For this review, take the finished solid that the model builds, in its own axes (mm). A direction names the side the tool comes from. Give positions to 0.01 mm unless a question says otherwise; leave off trailing zeros. Write each loop counter-clockwise with the first axis right and the second up, starting at its lowest first coordinate (ties: lowest second). Pieces come first, ordered by that corner, then holes. Notation, with made-up numbers: (89, 16.25) -> (126, 16.25) arc R22 cw to (126, 31.25) -> close; hole circle Ø11 at (-30.75, 64). An arc over 180 degrees is marked (long way). Write item = value, one per line.
```python
from build123d import *

# Parameters (mm, degrees)
SKETCH1_W          = 5
SKETCH1_H          = 36
SKETCH2_R          = 3.43154
CUT_EXTRUDE1_DEPTH = 0.5
SKETCH3_R          = 3.5
CUT_EXTRUDE2_DEPTH = 31.5
CUT_EXTRUDE3_REACH = 34.284
SKETCH4_R          = 1.5
CUT_EXTRUDE4_REACH = 38.688


with BuildPart() as part:
    # Sketch1 → Revolve1 (revolve)
    with BuildSketch(Plane.XY, mode=Mode.PRIVATE) as revolve1_sk:
        with Locations((2.5, 16.5)):
            Rectangle(SKETCH1_W, SKETCH1_H)
    revolve(revolve1_sk.sketch.rotate(Axis((0, 34.5, 0), (0, -1, 0)), 270), axis=Axis((0, 34.5, 0), (0, -1, 0)))

    # Sketch2 → Cut-Extrude1 (cut)
    with BuildSketch(Plane(origin=(0, 31.6, 0), x_dir=(1, 0, 0), z_dir=(0, 1, 0))):
        with Locations(Location((0, 0, 0), (0, 0, 90))):
            Circle(SKETCH2_R)
    extrude(amount=-CUT_EXTRUDE1_DEPTH, mode=Mode.SUBTRACT)

    # Sketch3 → Cut-Extrude2 (cut)
    with BuildSketch(Plane.XZ.offset(1.5)):
        with Locations(Location((0, 0, 0), (0, 0, 90))):
            Circle(SKETCH3_R)
    extrude(amount=-CUT_EXTRUDE2_DEPTH, mode=Mode.SUBTRACT)

    # Sketch4 → Cut-Extrude3 (cut, up to next)
    with BuildSketch(Plane.XZ.offset(-30), mode=Mode.PRIVATE) as cut_extrude3_sk1:
        with Locations(Location((0, 0, 0), (0, 0, 270))):
            Circle(SKETCH4_R)
    cut_extrude3_tool1 = extrude(cut_extrude3_sk1.sketch, amount=-CUT_EXTRUDE3_REACH, mode=Mode.PRIVATE) & part.part
    add(cut_extrude3_tool1.solids().sort_by_distance((0, 30, 0))[0], mode=Mode.SUBTRACT)

    # Sketch5 → Cut-Extrude4 (cut, up to next)
    with BuildSketch(Plane(origin=(0, 34.5, 0), x_dir=(-1, 0, 0), z_dir=(0, 1, 0)), mode=Mode.PRIVATE) as cut_extrude4_sk1:
        with BuildLine():
            Line((2.430309722, 1.842849602), (1.999275165, 1.739367361))
            ThreePointArc((1.999275165, 1.739367361), (1.931766863, 1.814049831), (1.861470643, 1.886114272))
            Line((1.861470643, 1.886114272), (1.991813569, 2.309800577))
            ThreePointArc((1.991813569, 2.309800577), (1.944143169, 2.35006539), (1.895659013, 2.389346544))
            Line((1.895659013, 2.389346544), (1.503901187, 2.181921452))
            ThreePointArc((1.503901187, 2.181921452), (1.419941007, 2.237469003), (1.333931574, 2.289787448))
            Line((1.333931574, 2.289787448), (1.354813039, 2.732577836))
            ThreePointArc((1.354813039, 2.732577836), (1.298626839, 2.75972251), (1.241897077, 2.785712054))
            Line((1.241897077, 2.785712054), (0.914031566, 2.487377393))
            ThreePointArc((0.914031566, 2.487377393), (0.818895035, 2.520299768), (0.722576679, 2.549584857))
            Line((0.722576679, 2.549584857), (0.632684622, 2.98365718))
            ThreePointArc((0.632684622, 2.98365718), (0.571513009, 2.995976115), (0.51010218, 3.007041032))
            Line((0.51010218, 3.007041032), (0.26672998, 2.636542265))
            ThreePointArc((0.26672998, 2.636542265), (0.166394877, 2.64477083), (0.065819633, 2.649182473))
            Line((0.065819633, 2.649182473), (-0.129197696, 3.047262371))
            ThreePointArc((-0.129197696, 3.047262371), (-0.191511085, 3.043981522), (-0.253744312, 3.039426562))
            Line((-0.253744312, 3.039426562), (-0.397331231, 2.620043491))
            ThreePointArc((-0.397331231, 2.620043491), (-0.496560484, 2.603061214), (-0.595073102, 2.582322211))
            Line((-0.595073102, 2.582322211), (-0.882962048, 2.919396859))
            ThreePointArc((-0.882962048, 2.919396859), (-0.942501833, 2.900722375), (-1.001647117, 2.880833743))
            Line((-1.001647117, 2.880833743), (-1.03642666, 2.438917747))
            ThreePointArc((-1.03642666, 2.438917747), (-1.128315123, 2.397791689), (-1.218575206, 2.353205148))
            Line((-1.218575206, 2.353205148), (-1.581246647, 2.608094906))
            ThreePointArc((-1.581246647, 2.608094906), (-1.634271725, 2.575200173), (-1.686612749, 2.541227545))
            Line((-1.686612749, 2.541227545), (-1.61039959, 2.104545832))
            ThreePointArc((-1.61039959, 2.104545832), (-1.689173573, 2.041860093), (-1.765509747, 1.976227551))
            Line((-1.765509747, 1.976227551), (-2.180175704, 2.132916759))
            ThreePointArc((-2.180175704, 2.132916759), (-2.223354314, 2.087868673), (-2.2656023, 2.041946674))
            Line((-2.2656023, 2.041946674), (-2.083185191, 1.637937563))
            ThreePointArc((-2.083185191, 1.637937563), (-2.143895035, 1.557630919), (-2.201510819, 1.475076308))
            Line((-2.201510819, 1.475076308), (-2.642116303, 1.523719607))
            ThreePointArc((-2.642116303, 1.523719607), (-2.672735374, 1.469348706), (-2.702235725, 1.414362784))
            Line((-2.702235725, 1.414362784), (-2.425076605, 1.068411652))
            ThreePointArc((-2.425076605, 1.068411652), (-2.463907688, 0.975530065), (-2.499182869, 0.881240596))
            Line((-2.499182869, 0.881240596), (-2.938043018, 0.818781548))
            ThreePointArc((-2.938043018, 0.818781548), (-2.954178641, 0.758504156), (-2.969077742, 0.697909279))
            Line((-2.969077742, 0.697909279), (-2.614591538, 0.431753508))
            ThreePointArc((-2.614591538, 0.431753508), (-2.629103958, 0.332133069), (-2.639822068, 0.232033297))
            Line((-2.639822068, 0.232033297), (-3.049361685, 0.062396433))
            ThreePointArc((-3.049361685, 0.062396433), (-3.05, 0), (-3.049361685, -0.062396433))
            Line((-3.049361685, -0.062396433), (-2.639822068, -0.232033297))
            ThreePointArc((-2.639822068, -0.232033297), (-2.629103958, -0.332133069), (-2.614591538, -0.431753508))
            Line((-2.614591538, -0.431753508), (-2.969077742, -0.697909279))
            ThreePointArc((-2.969077742, -0.697909279), (-2.954178641, -0.758504156), (-2.938043018, -0.818781548))
            Line((-2.938043018, -0.818781548), (-2.499182869, -0.881240596))
            ThreePointArc((-2.499182869, -0.881240596), (-2.463907688, -0.975530065), (-2.425076605, -1.068411652))
            Line((-2.425076605, -1.068411652), (-2.702235725, -1.414362784))
            ThreePointArc((-2.702235725, -1.414362784), (-2.672735374, -1.469348706), (-2.642116303, -1.523719607))
            Line((-2.642116303, -1.523719607), (-2.201510819, -1.475076308))
            ThreePointArc((-2.201510819, -1.475076308), (-2.143895035, -1.557630919), (-2.083185191, -1.637937563))
            Line((-2.083185191, -1.637937563), (-2.2656023, -2.041946674))
            ThreePointArc((-2.2656023, -2.041946674), (-2.223354314, -2.087868673), (-2.180175704, -2.132916759))
            Line((-2.180175704, -2.132916759), (-1.765509747, -1.976227551))
            ThreePointArc((-1.765509747, -1.976227551), (-1.689173573, -2.041860093), (-1.61039959, -2.104545832))
            Line((-1.61039959, -2.104545832), (-1.686612749, -2.541227545))
            ThreePointArc((-1.686612749, -2.541227545), (-1.634271725, -2.575200173), (-1.581246647, -2.608094906))
            Line((-1.581246647, -2.608094906), (-1.218575206, -2.353205148))
            ThreePointArc((-1.218575206, -2.353205148), (-1.128315123, -2.397791689), (-1.03642666, -2.438917747))
            Line((-1.03642666, -2.438917747), (-1.001647117, -2.880833743))
            ThreePointArc((-1.001647117, -2.880833743), (-0.942501833, -2.900722375), (-0.882962048, -2.919396859))
            Line((-0.882962048, -2.919396859), (-0.595073102, -2.582322211))
            ThreePointArc((-0.595073102, -2.582322211), (-0.496560484, -2.603061214), (-0.397331231, -2.620043491))
            Line((-0.397331231, -2.620043491), (-0.253744312, -3.039426562))
            ThreePointArc((-0.253744312, -3.039426562), (-0.191511085, -3.043981522), (-0.129197696, -3.047262371))
            Line((-0.129197696, -3.047262371), (0.065819633, -2.649182473))
            ThreePointArc((0.065819633, -2.649182473), (0.166394877, -2.64477083), (0.26672998, -2.636542265))
            Line((0.26672998, -2.636542265), (0.51010218, -3.007041032))
            ThreePointArc((0.51010218, -3.007041032), (0.571513009, -2.995976115), (0.632684622, -2.98365718))
            Line((0.632684622, -2.98365718), (0.722576679, -2.549584857))
            ThreePointArc((0.722576679, -2.549584857), (0.818895035, -2.520299768), (0.914031566, -2.487377393))
            Line((0.914031566, -2.487377393), (1.241897077, -2.785712054))
            ThreePointArc((1.241897077, -2.785712054), (1.298626839, -2.75972251), (1.354813039, -2.732577836))
            Line((1.354813039, -2.732577836), (1.333931574, -2.289787448))
            ThreePointArc((1.333931574, -2.289787448), (1.419941007, -2.237469003), (1.503901187, -2.181921452))
            Line((1.503901187, -2.181921452), (1.895659013, -2.389346544))
            ThreePointArc((1.895659013, -2.389346544), (1.944143169, -2.35006539), (1.991813569, -2.309800577))
            Line((1.991813569, -2.309800577), (1.861470643, -1.886114272))
            ThreePointArc((1.861470643, -1.886114272), (1.931766863, -1.814049831), (1.999275165, -1.739367361))
            Line((1.999275165, -1.739367361), (2.430309722, -1.842849602))
            ThreePointArc((2.430309722, -1.842849602), (2.467501833, -1.792745019), (2.503661128, -1.741890052))
            Line((2.503661128, -1.741890052), (2.272046665, -1.3639296))
            ThreePointArc((2.272046665, -1.3639296), (2.322212702, -1.276647236), (2.369027332, -1.187522421))
            Line((2.369027332, -1.187522421), (2.812255133, -1.180559643))
            ThreePointArc((2.812255133, -1.180559643), (2.835818282, -1.122779886), (2.858194451, -1.06453017))
            Line((2.858194451, -1.06453017), (2.539861639, -0.756044214))
            ThreePointArc((2.539861639, -0.756044214), (2.566745377, -0.659028201), (2.589924799, -0.561061081))
            Line((2.589924799, -0.561061081), (3.01749621, -0.444090779))
            ThreePointArc((3.01749621, -0.444090779), (3.025949839, -0.382266362), (3.033136904, -0.320281942))
            Line((3.033136904, -0.320281942), (2.648087766, -0.100653791))
            ThreePointArc((2.648087766, -0.100653791), (2.65, 0), (2.648087766, 0.100653791))
            Line((2.648087766, 0.100653791), (3.033136904, 0.320281942))
            ThreePointArc((3.033136904, 0.320281942), (3.025949839, 0.382266362), (3.01749621, 0.444090779))
            Line((3.01749621, 0.444090779), (2.589924799, 0.561061081))
            ThreePointArc((2.589924799, 0.561061081), (2.566745377, 0.659028201), (2.539861639, 0.756044214))
            Line((2.539861639, 0.756044214), (2.858194451, 1.06453017))
            ThreePointArc((2.858194451, 1.06453017), (2.835818282, 1.122779886), (2.812255133, 1.180559643))
            Line((2.812255133, 1.180559643), (2.369027332, 1.187522421))
            ThreePointArc((2.369027332, 1.187522421), (2.322212702, 1.276647236), (2.272046665, 1.3639296))
            Line((2.272046665, 1.3639296), (2.503661128, 1.741890052))
            ThreePointArc((2.503661128, 1.741890052), (2.467501833, 1.792745019), (2.430309722, 1.842849602))
        make_face()
    cut_extrude4_tool1 = extrude(cut_extrude4_sk1.sketch, amount=-CUT_EXTRUDE4_REACH, mode=Mode.PRIVATE) & part.part
    add(cut_extrude4_tool1.solids().sort_by_distance((0, 34.5, 0))[0], mode=Mode.SUBTRACT)


solid = part.part
```
(1) Take a section at B-B (x = 4). Write out the cut boundary in (y, z).
Answers below:
outline = (-1.5, -3) -> (34.5, -3) -> (34.5, 3) -> (-1.5, 3) -> close
(2) Take a section at A-A (y = 18). Write out the cut boundary in (x, z), plus the area to 3 significant figures.
Answers below:
outline = circle Ø10 at (0, 0); hole circle Ø7 at (0, 0)
area = 40.1 mm^2
(3) Tool access review of faces 5 (the face through (3.417, 14.03, -0.759)), 6 (the face through (-3.3, -1.5, 2.2)), 7 (the face through (0.7, 31.1, -1.5)): name each direction out of +Z, -Z, +X, -X, +Y, -Y from which nothing blocks a thin tool from reaching the whole face with its end or side.
Answers below:
face_5 = -Y
face_6 = +Z, -Z, +X, -X, -Y
face_7 = none
(4) For pin 1 (4 mm diameter, centred on x = 0, z = 0, fed in from -Y); pin 2 (4 mm diameter, centred on x = 0, z = 0, fed in from +Y); pin 3 (5 mm diameter, centred on y = 3, z = 3.5, fed in from -X), all flat-tipped, find the tip position at first contact; note any pin that passes through.
Answers below:
pin_1 = 30
pin_2 = 31.1
pin_3 = -4.9
(5) The part is to be moulded in two halves that separate along X. For faces 1 (the face through (3, 31.6, 1)), 2 (the face through (-2.2, 34.5, 2.2)), 3 (the face through (0, 30, 2)), 4 (the face through (-4.88, 16.75, 1.08)), say which applies: released by +X, released by -X, zero draft, split by the parting line, or undercut.
Answers below:
face_1 = undercut
face_2 = zero draft
face_3 = undercut
face_4 = split by the parting line
(6) To check wall thickness, follow probe 1 along X at (y, z) = (13, 0); probe 2 along Y at (x, z) = (-2, -2.5); probe 3 along X at (y, z) = (30.7, 0). State the ranges of each line that lie inside material, in increasing order.
Answers below:
probe_1 = -5 to -3.5, 3.5 to 5
probe_2 = 30 to 31.1, 31.6 to 34.5
probe_3 = -5 to -1.5, 1.5 to 5
